from build123d import *

# Parameters (mm, degrees)
F1_DEPTH = 10


with BuildPart() as f1:
    # F0 (on Front) → F1 (new body)
    with BuildSketch(Plane.XZ):
        with BuildLine():
            Line((-100, 0), (-20, 0))
            ThreePointArc((-20, 0), (0, 20), (-20, 40))
            Line((-20, 40), (-100, 40))
            Line((-100, 40), (-100, 0))
        make_face()
        with BuildLine():
            ThreePointArc((-70.317542, 17.5), (-90, 20), (-70.317542, 22.5))
            Line((-70.317542, 22.5), (-68, 22.5))
            Line((-68, 22.5), (-68, 20))
            Line((-68, 20), (-68, 17.5))
            Line((-68, 17.5), (-70.317542, 17.5))
        make_face(mode=Mode.SUBTRACT)
    extrude(amount=F1_DEPTH)


solid = f1.part
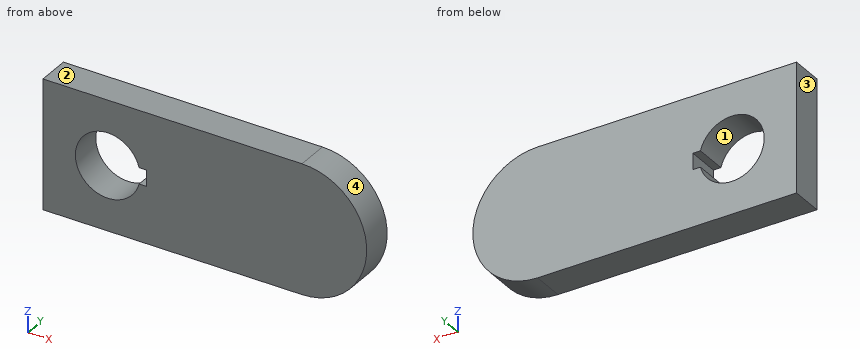
Geometry: final body of the model. Coordinates: model frame, mm. Face numbers are marked on the shaded views. Give positions to 0.01 mm unless a question says otherwise; leave off trailing zeros. Order: outer loops, then holes, each group sorted by start corner. A loop starts at its lowest first (then second) coordinate and runs counter-clockwise, first axis right, second up. Notation, with made-up numbers: (49.5, 65.25) -> (60.5, 65.25) arc R12 cw to (60.5, 81.25) -> close; hole circle Ø4 at (57, 51). An arc over 180 degrees is marked (long way). Answer as a JSON object with one key per item and string values.
Q1. Section B-B (y = -8.75). Output: boundary loops of the cut face in (x, z), plus the area to 3 significant figures.
Entries:
{"outline": "(-100, 0) -> (-20, 0) arc R20 ccw to (-20, 40) -> (-100, 40) -> close; hole (-70.32, 17.5) -> (-68, 17.5) -> (-68, 22.5) -> (-70.32, 22.5) arc R10 ccw (long way) to start", "area": "3,500 mm^2"}
Q2. Section D-D (x = -6.5). Output: boundary loops of the cut face in (y, z).
Entries:
{"outline": "(-10, 5.24) -> (0, 5.24) -> (0, 34.76) -> (-10, 34.76) -> close"}
Q3. Section C-C (z = 28.5). Output: boundary loops of the cut face in (x, y).
Entries:
{"outline": "(-100, -10) -> (-85.27, -10) -> (-85.27, 0) -> (-100, 0) -> close; (-74.73, -10) -> (-1.9, -10) -> (-1.9, 0) -> (-74.73, 0) -> close"}
Q4. Draft query along Z for the marked faces 1, 2, 3 and 4. Return one class per face: released by +Z, released by -Z, zero draft, split by the parting line, or undercut.
Entries:
{"face 1": "undercut", "face 2": "released by +Z", "face 3": "zero draft", "face 4": "split by the parting line"}
Q5. First-contact query: pin 1 (16 mm diameter, centred on x = -80, z = 20, fed in from -Y). Flat tip, straight axial feed; report the tip coordinate or a pass-through.
Entries:
{"pin 1": "passes through"}
Q6. Section A-A (x = -80). Output: boundary loops of the cut face in (y, z), plus the area to 3 significant figures.
Entries:
{"outline": "(-10, 0) -> (0, 0) -> (0, 10) -> (-10, 10) -> close; (-10, 30) -> (0, 30) -> (0, 40) -> (-10, 40) -> close", "area": "200 mm^2"}
Q7. Material intervals for probe 1 along X at (y, z) = (-6.25, 20); probe 2 along Z at (x, y) = (-80, -3.75); probe 3 along Z at (x, y) = (-83, -1.25), sorted ascending.
Entries:
{"probe 1": "x = -100 to -90, -68 to 0", "probe 2": "z = 0 to 10, 30 to 40", "probe 3": "z = 0 to 10.46, 29.54 to 40"}
